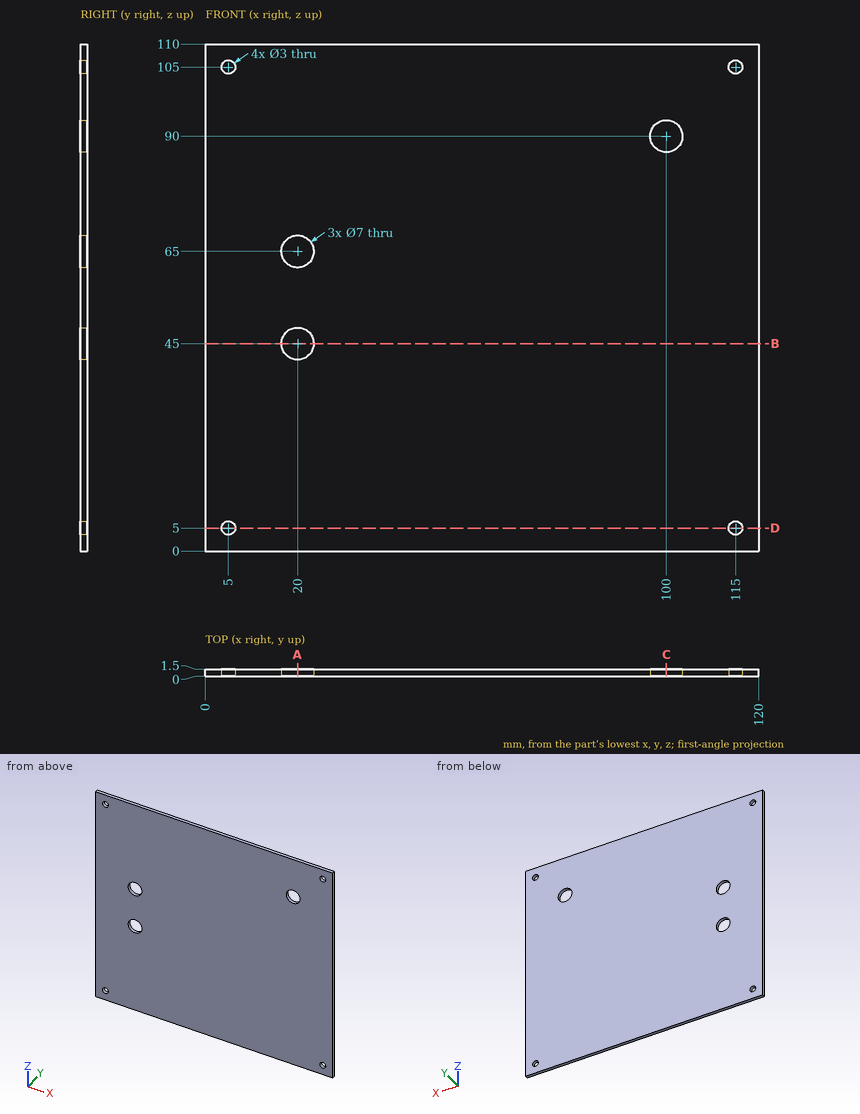
Drawing for the job (mm, zero at the part's lowest x, y, z). Give positions to 0.01 mm unless a question says otherwise; leave off trailing zeros. Order: outer loops, then holes, each group sorted by start corner. A loop starts at its lowest first (then second) coordinate and runs counter-clockwise, first axis right, second up. Notation, with made-up numbers: (69.25, 0.5) - (108.25, 0.5) arc R17 ccw to (108.25, 8.5) - close; hole circle Ø4 at (58, 32). An arc over 180 degrees is marked (long way). Use one line per item in the form item = value.
Item 1: Pin check, flat tips, straight feed: pin 1 Ø6.5 at (x, z) = (100, 90) entering from -Y; pin 2 Ø3.5 at (x, z) = (115, 5) entering from +Y. Stop position of each tip, or through.
Solution:
pin_1 = through
pin_2 = 1.5
Item 2: Slice it at D-D on z = 5. Give the cut face in (x, y), and give its area (3 significant figures).
Solution:
outline = (0, 0) - (3.5, 0) - (3.5, 1.5) - (0, 1.5) - close; (6.5, 0) - (113.5, 0) - (113.5, 1.5) - (6.5, 1.5) - close; (116.5, 0) - (120, 0) - (120, 1.5) - (116.5, 1.5) - close
area = 171 mm2
Item 3: Slice it at C-C on x = 100. Give the cut face in (y, z).
Solution:
outline = (0, 0) - (1.5, 0) - (1.5, 86.5) - (0, 86.5) - close; (0, 93.5) - (1.5, 93.5) - (1.5, 110) - (0, 110) - close
Item 4: Slice it at A-A on x = 20. Give the cut face in (y, z), and give its area (3 significant figures).
Solution:
outline = (0, 0) - (1.5, 0) - (1.5, 41.5) - (0, 41.5) - close; (0, 48.5) - (1.5, 48.5) - (1.5, 61.5) - (0, 61.5) - close; (0, 68.5) - (1.5, 68.5) - (1.5, 110) - (0, 110) - close
area = 144 mm2
Item 5: Slice it at B-B on z = 45. Give the cut face in (x, y).
Solution:
outline = (0, 0) - (16.5, 0) - (16.5, 1.5) - (0, 1.5) - close; (23.5, 0) - (120, 0) - (120, 1.5) - (23.5, 1.5) - close
Item 6: Probe probe 1 along X at (y, z) = (0.6, 105); probe 2 along X at (y, z) = (0.45, 65). List the from-to ranges inside material, lowest first. Write a range as from..to.
Solution:
probe_1 = 0..3.5, 6.5..113.5, 116.5..120
probe_2 = 0..16.5, 23.5..120
